Input: part model. Units: mm. Frame: model coordinates. A direction names the side the tool comes from. Coordinates: 2 decimals unless noted, no trailing zeros. Loops run counter-clockwise (first coordinate to the right, second up) from the corner with the lowest first, then second, coordinate; pieces in that order, holes last.
Item 1: Section D-D on y = -0.25. Return loops of the section in (x, z), and give its area (3 significant figures).
Item 2: Section B-B on z = 3. Return loops of the section in (x, y), and give its area (3 significant figures).
Item 3: Section C-C on x = 0. Return loops of the section in (y, z), and give its area (3 significant figures).
Item 4: Reachability of faces 1 (the cylindrical face through (-4.59, 11.14, 4.24)), 2 (the flat face through (0, 12, 8)), 3 (the flat face through (0, 10.1, 7)) from +Z, -Z, +X, -X, +Y, -Y: full face, straight path, thin tool, end or side. Return the list, or none.
Item 5: Ray query, line 1 along X through (y, z) = (10.5, 2); line 2 along Z through (x, y) = (-4.75, 10.35); line 3 along Z through (x, y) = (4.75, 9.95). Return the intervals inside material, ascending.
Item 6: Contact query for flat-ended pins moving along their axis: P1, Ø1, axis at x = -3.5, z = 7.5, coming from the -Y side; P2, Ø5, axis at x = 2, y = 1.5, coming from the +Z side; P3, Ø4, axis at x = -4.75, z = 3, coming from the -Y side. Output: stop coordinate, or through.
Item 7: Pull-direction query (X, two-part tool) for faces 4 (the cylindrical face through (5.671, 11.142, 3.845)), 5 (the flat face through (0, 6, 0)), 6 (the flat face through (8.214, 4.015, 2.958)); classes: released by +X, released by -X, zero draft, split by the parting line, or undercut.
Item 8: Section A-A on y = 11.25. Return loops of the section in (x, z), and give its area (3 significant figures).
```python
from build123d import *

# Parameters (mm, degrees)
F0_R     = 2.75
F1_DEPTH = 6
F0_W     = 20
F0_H     = 4
F2_DEPTH = 8
F3_R     = 1.25
F4_DEPTH = 6
F5_R     = 2


with BuildPart() as f1:
    # F0 (on Top) → F1 (new body)
    with BuildSketch(Plane.XY):
        with BuildLine():
            Line((-10, 10.1), (-6.476664, -1.9014))
            ThreePointArc((-6.476664, -1.9014), (0, -6.75), (6.476664, -1.9014))
            Line((6.476664, -1.9014), (10, 10.1))
            Line((10, 10.1), (-10, 10.1))
        make_face()
        Circle(F0_R, mode=Mode.SUBTRACT)
    extrude(amount=F1_DEPTH)

    # F0 (on Top) → F2 (join)
    with BuildSketch(Plane.XY):
        with Locations((0, 12.1)):
            Rectangle(F0_W, F0_H)
    extrude(amount=F2_DEPTH)

    # F3 (on face) → F4 (cut)
    with BuildSketch(Plane(origin=(0, 14.1, 0), x_dir=(-1, 0, 0), z_dir=(0, 1, 0))):
        with Locations((-4.75, 3)):
            Circle(F3_R)
        with Locations((4.75, 3)):
            Circle(F3_R)
    extrude(amount=-F4_DEPTH, mode=Mode.SUBTRACT)

    # F5
    f5_edges = [f1.edges().sort_by_distance(p)[0] for p in [
        (-10, 12.1, 8),
        (10, 12.1, 8),
    ]]
    fillet(f5_edges, radius=F5_R)


solid = f1.part
```
Results found:
1. outline: (-6.96, 0) - (-2.74, 0) - (-2.74, 6) - (-6.96, 6) - close; (2.74, 0) - (6.96, 0) - (6.96, 6) - (2.74, 6) - close
1. area: 50.7 mm2
2. outline: (-10, 10.1) - (-6.48, -1.9) arc R6.75 ccw to (6.48, -1.9) - (10, 10.1) - (10, 14.1) - (6, 14.1) - (6, 8.1) - (3.5, 8.1) - (3.5, 14.1) - (-3.5, 14.1) - (-3.5, 8.1) - (-6, 8.1) - (-6, 14.1) - (-10, 14.1) - close; hole circle Ø5.5 at (0, 0)
2. area: 270 mm2
3. outline: (-6.75, 0) - (-2.75, 0) - (-2.75, 6) - (-6.75, 6) - close; (2.75, 0) - (14.1, 0) - (14.1, 8) - (10.1, 8) - (10.1, 6) - (2.75, 6) - close
3. area: 100 mm2
4. face 1: +Y
4. face 2: +Z, +X, -X, +Y, -Y
4. face 3: +Z, +X, -X, -Y
5. line 1: x = -10 to -5.5, -4 to 4, 5.5 to 10
5. line 2: z = 0 to 1.75, 4.25 to 8
5. line 3: z = 0 to 1.75, 4.25 to 6
6. P1: stops at y = 10.1
6. P2: stops at z = 6
6. P3: stops at y = -6.16
7. face 4: undercut
7. face 5: zero draft
7. face 6: released by +X
8. outline: (-10, 0) - (10, 0) - (10, 6) arc R2 ccw to (8, 8) - (-8, 8) arc R2 ccw to (-10, 6) - close; hole circle Ø2.5 at (-4.75, 3); hole circle Ø2.5 at (4.75, 3)
8. area: 148 mm2
